from build123d import *

# Parameters (mm, degrees)
CROQUIS1_R              = 3
CROQUIS1_R_2            = 6
SALIENTE_EXTRUIR1_DEPTH = 6


with BuildPart() as part:
    # Croquis1 → Saliente-Extruir1 (new body)
    with BuildSketch(Plane.XY):
        with BuildLine():
            ThreePointArc((0, -6), (2.10674065, -5.617975065), (3.945205479, -4.520547945))
            ThreePointArc((3.945205479, -4.520547945), (5.462198865, -2.482817666), (6, 0))
            ThreePointArc((6, 0), (4.242640687, 4.242640687), (0, 6))
            ThreePointArc((0, 6), (-4.242640687, 4.242640687), (-6, 0))
            ThreePointArc((-6, 0), (-4.242640687, -4.242640687), (0, -6))
        make_face()
        Circle(CROQUIS1_R, mode=Mode.SUBTRACT)
        with BuildLine():
            ThreePointArc((14.287671233, 4.505603985), (15.551832387, 6.203712551), (16, 8.272727273))
            Line((16, 8.272727273), (16, 106.727272727))
            ThreePointArc((16, 106.727272727), (15.551832387, 108.796287449), (14.287671233, 110.494396015))
            Line((14.287671233, 110.494396015), (3.945205479, 119.520547945))
            ThreePointArc((3.945205479, 119.520547945), (5.462198865, 117.482817666), (6, 115))
            ThreePointArc((6, 115), (4.242640687, 110.757359313), (0, 109))
            Line((0, 109), (1, 109))
            ThreePointArc((1, 109), (4.535533906, 107.535533906), (6, 104))
            Line((6, 104), (6, 11))
            ThreePointArc((6, 11), (4.535533906, 7.464466094), (1, 6))
            Line((1, 6), (0, 6))
            ThreePointArc((0, 6), (4.242640687, 4.242640687), (6, 0))
            ThreePointArc((6, 0), (5.462198865, -2.482817666), (3.945205479, -4.520547945))
            Line((3.945205479, -4.520547945), (14.287671233, 4.505603985))
        make_face()
        with Locations((0, 115)):
            Circle(CROQUIS1_R_2)
        with Locations((0, 115)):
            Circle(CROQUIS1_R, mode=Mode.SUBTRACT)
    extrude(amount=SALIENTE_EXTRUIR1_DEPTH)


solid = part.part
For this review, take the finished solid that the model builds, in its own axes (mm). A direction names the side the tool comes from. Round coordinates to 2 decimals unless told otherwise and drop trailing zeros. Loops run counter-clockwise (first coordinate to the right, second up) from the corner with the lowest first, then second, coordinate; pieces in that order, holes last. Notation, with made-up numbers: (23.5, 53) - (58.5, 53) arc R18 cw to (58.5, 72) - close; hole circle Ø1 at (-1, 7.5). An arc over 180 degrees is marked (long way). Put each result on its own line as item: value. Start each with the question number.
1. Consider section C-C on y = 115. State the section outline as (x, z) points (3 decimals).
2. Insertion check: P1, Ø0.5, axis at x = 0.5, z = 4, coming from the +Y side; P2, Ø2, axis at x = 8, z = 1, coming from the -Y side; P3, Ø1.5, axis at y = 30.5, z = 3, coming from the -X side; P4, Ø10, axis at x = -0.5, y = 70.5, coming from the +Z side (1 decimal). Each pin has a flat end and moves straight along its axis. Give the tip position at first contact, or say it passes through.
3. Consider section B-B on x = -1.75. State the section outline as (y, z) points.
4. Consider section D-D on y = 46.5. State the section outline as (x, z) points.
5. Mouldability with a two-part tool opening along Y and no side actions: class faces 3 (the cylindrical face through (15.564, 108.769, 2.958)), 4 (the cylindrical face through (4, 108, 3)), 5 (the flat face through (16, 57, 3)), 6 (the flat face through (9.044, -0.071, 2.958)) as +Y half, -Y half, draft (parallel to the pull), parting line (faces both ways), or undercut.
6. For faces 1 (the cylindrical face through (0, 118, 3)), 2 (the flat face through (6, 58, 3)), list the 3-axis set-ups (+Z, -Z, +X, -X, +Y, -Y) from which the entire face can be reached by the end or side of a thin tool; tool diameter is ignored.
7. For probe 1 along Y at (x, z) = (0.75, 5.7); probe 2 along X at (y, z) = (36.5, 3.15); probe 3 along Y at (x, z) = (5.5, 3.6), list the stretches that pass through material, from the lowest coordinate up. Write a range as [from, to].
8. Consider section A-A on z = 0.95. State the section outline as (x, y) points, plus the area to 3 significant figures.
Result sheet:
1. outline: (-6, 0) - (-3, 0) - (-3, 6) - (-6, 6) - close; (3, 0) - (9.125, 0) - (9.125, 6) - (3, 6) - close
2. P1: y = 120.99
2. P2: y = -1.85
2. P3: x = 6
2. P4: through
3. outline: (-5.74, 0) - (-2.44, 0) - (-2.44, 6) - (-5.74, 6) - close; (2.44, 0) - (5.74, 0) - (5.74, 6) - (2.44, 6) - close; (109.26, 0) - (112.56, 0) - (112.56, 6) - (109.26, 6) - close; (117.44, 0) - (120.74, 0) - (120.74, 6) - (117.44, 6) - close
4. outline: (6, 0) - (16, 0) - (16, 6) - (6, 6) - close
5. face 3: +Y half
5. face 4: undercut
5. face 5: draft
5. face 6: -Y half
6. face 1: +Z, -Z
6. face 2: +Z, -Z, -X
7. probe 1: [-5.95, -2.9], [2.9, 6], [109, 112.1], [117.9, 120.95]
7. probe 2: [6, 16]
7. probe 3: [-3.16, 8.82], [106.18, 118.16]
8. outline: (0, 6) arc R6 ccw (long way) to (3.95, -4.52) - (14.29, 4.51) arc R5 ccw to (16, 8.27) - (16, 106.73) arc R5 ccw to (14.29, 110.49) - (3.95, 119.52) arc R6 ccw (long way) to (0, 109) - (1, 109) arc R5 cw to (6, 104) - (6, 11) arc R5 cw to (1, 6) - close; hole circle Ø6 at (0, 0); hole circle Ø6 at (0, 115)
8. area: 1,310 mm^2
